from build123d import *

# Parameters (mm, degrees)
SKETCH3_R           = 10
SKETCH3_R_2         = 9
SKETCH3_R_3         = 8
SKETCH3_R_4         = 5
BOSS_EXTRUDE1_DEPTH = 5
CUT_EXTRUDE1_DEPTH  = 5
CIRPATTERN1_COUNT   = 12
SKETCH3_3_R         = 5
CUT_EXTRUDE3_DEPTH  = 5


with BuildPart() as part:
    # Sketch3 → Boss-Extrude1 (new body)
    # profile 1 of 4: a face of its own
    with BuildSketch(Plane(origin=(0, 0, 0), x_dir=(0, 0, -1), z_dir=(1, 0, 0))):
        Circle(SKETCH3_R)
        Circle(SKETCH3_R_2, mode=Mode.SUBTRACT)
    # profile 2 of 4: a face of its own
    with BuildSketch(Plane(origin=(0, 0, 0), x_dir=(0, 0, -1), z_dir=(1, 0, 0))):
        Circle(SKETCH3_R_2)
        Circle(SKETCH3_R_3, mode=Mode.SUBTRACT)
    # profile 3 of 4: a face of its own
    with BuildSketch(Plane(origin=(0, 0, 0), x_dir=(0, 0, -1), z_dir=(1, 0, 0))):
        Circle(SKETCH3_R_3)
        Circle(SKETCH3_R_4, mode=Mode.SUBTRACT)
    # profile 4 of 4: a face of its own
    with BuildSketch(Plane(origin=(0, 0, 0), x_dir=(0, 0, -1), z_dir=(1, 0, 0))):
        Circle(SKETCH3_R_4)
    extrude(amount=BOSS_EXTRUDE1_DEPTH)

    # Gear_Profile → Cut-Extrude1 (cut)
    with BuildSketch(Plane.ZY):
        with BuildLine():
            ThreePointArc((-0.410698141, 7.989450985), (-0.205416799, 7.997362311), (0, 8))
            Line((0, 8), (0, 10))
            ThreePointArc((0, 10), (-0.973914923, 9.952461491), (-1.938570153, 9.810297945))
            Line((-1.938570153, 9.810297945), (-1.595423995, 9.401352278))
            Line((-1.595423995, 9.401352278), (-0.410698141, 7.989450985))
        make_face()
        with BuildLine():
            ThreePointArc((-1.595423995, 9.401352278), (-1.193917878, 8.71367126), (-1.044209538, 7.931558891))
            ThreePointArc((-1.044209538, 7.931558891), (-0.728029506, 7.966804443), (-0.410698141, 7.989450985))
            Line((-0.410698141, 7.989450985), (-1.595423995, 9.401352278))
        make_face()
        with BuildLine():
            ThreePointArc((0, 8), (0.523225034, 7.982871386), (1.044209538, 7.931558891))
            ThreePointArc((1.044209538, 7.931558891), (1.311715504, 8.977395553), (2.017271047, 9.794417671))
            ThreePointArc((2.017271047, 9.794417671), (1.013859775, 9.948471659), (0, 10))
            Line((0, 10), (0, 8))
        make_face()
    cut_extrude1 = extrude(amount=-CUT_EXTRUDE1_DEPTH, mode=Mode.SUBTRACT)

    # CirPattern1: Cut-Extrude1 ×12 about axis
    cirpattern1_axis = Axis((0, 0, 0), (1, 0, 0))
    for i in range(1, CIRPATTERN1_COUNT):
        add(cut_extrude1.rotate(cirpattern1_axis, i * 360 / CIRPATTERN1_COUNT), mode=Mode.SUBTRACT)

    # Sketch3_3 → Cut-Extrude3 (cut)
    with BuildSketch(Plane(origin=(0, 0, 0), x_dir=(0, 0, -1), z_dir=(1, 0, 0))):
        Circle(SKETCH3_3_R)
    extrude(amount=CUT_EXTRUDE3_DEPTH, mode=Mode.SUBTRACT)


solid = part.part
The listing builds one solid part. Answer for the finished solid, in the listing's coordinates (mm). Round coordinates to 2 decimals unless told otherwise and drop trailing zeros. Write each question's results on one line, items separated by ' | '. Start each with the question number.
Q1. Each of these flat-tipped pins is pushed along its axis until it touches: pin 1 (2 mm diameter, centred on x = 2.5, z = 3, fed in from +Y); pin 2 (1.5 mm diameter, centred on x = 2.5, y = 3, fed in from -Z). Where does it stop, or does it pass through?
Q2. The mould has two halves that part along Y. Classify faces 1 (the cylindrical face through (2.465, -2.558, -9.667)), 2 (the cylindrical face through (2.465, -5.399, -6.956)), 3 (the cylindrical face through (2.465, 2.558, 9.667)), 4 (the cylindrical face through (2.46, -5.61, 7.11)): pulls with the +Y half, pulls with the -Y half, needs draft (parallel to the pull), parting line crosses it, or undercut.
Q3. Straight lines are drawn through the part: probe 1 along Y at (x, z) = (4, -6.75); probe 2 along Z at (x, y) = (3.9, -2.5); probe 3 along Z at (x, y) = (0.65, -3.75). For each, find the intervals that lie inside material, in ascending order. Write a range as from..to.
Worked answers:
1) pin 1: stops at y = 9.79 | pin 2: stops at z = -9.74
2) face 1: pulls with the -Y half | face 2: undercut | face 3: pulls with the +Y half | face 4: undercut
3) probe 1: y = -7.38..-5.18, -4.29..4.29, 5.18..7.38 | probe 2: z = -9.68..-4.33, 4.33..9.68 | probe 3: z = -7.07..-3.31, 3.31..7.07
